```python
from build123d import *

# Parameters (mm, degrees)
F0_W     = 140
F0_H     = 157.3
F0_W_2   = 5.7
F0_H_2   = 42
F0_W_3   = 42
F0_H_3   = 5.7
F0_W_4   = 9.225
F0_H_4   = 11.7
F0_W_5   = 20.361793
F0_H_5   = 125.9
F1_DEPTH = 5.8


with BuildPart() as f1:
    # F0 (on Right) → F1 (new body)
    with BuildSketch(Plane.YZ):
        Rectangle(F0_W, F0_H)
        with Locations((-62.15, -41.3)):
            Rectangle(F0_W_2, F0_H_2, mode=Mode.SUBTRACT)
        with Locations((-32.65, -70.8)):
            Rectangle(F0_W_3, F0_H_3, mode=Mode.SUBTRACT)
        with Locations((-25.8, -41.3)):
            Rectangle(F0_W_2, F0_H_2, mode=Mode.SUBTRACT)
        with Locations((29.475, -70.8)):
            Rectangle(F0_W_3, F0_H_3, mode=Mode.SUBTRACT)
        with Locations((60.0875, -61.45)):
            Rectangle(F0_W_4, F0_H_4, mode=Mode.SUBTRACT)
        with BuildLine():
            ThreePointArc((18.376166, -14.378899), (17.848958, -15.651691), (16.576166, -16.178899))
            Line((16.576166, -16.178899), (2.137455, -16.178901))
            ThreePointArc((2.137455, -16.178901), (0.864663, -15.651693), (0.337455, -14.378901))
            Line((0.337455, -14.378901), (0.337455, 5.028724))
            ThreePointArc((0.337455, 5.028724), (0.864663, 6.301516), (2.137455, 6.828724))
            Line((2.137455, 6.828724), (16.576166, 6.828722))
            ThreePointArc((16.576166, 6.828722), (17.848958, 6.301515), (18.376166, 5.028722))
            Line((18.376166, 5.028722), (18.376166, -1.151716))
            Line((18.376166, -1.151716), (13.94928, -1.151716))
            Line((13.94928, -1.151716), (13.94928, 3.184902))
            Line((13.94928, 3.184902), (4.764341, 3.184902))
            Line((4.764341, 3.184902), (4.764341, -12.535078))
            Line((4.764341, -12.535078), (13.94928, -12.535078))
            Line((13.94928, -12.535078), (13.94928, -7.927517))
            Line((13.94928, -7.927517), (18.376166, -7.927517))
            Line((18.376166, -7.927517), (18.376166, -14.378899))
        make_face(mode=Mode.SUBTRACT)
        Polygon((25.663247, -16.178899), (21.146094, -16.118674), (28.915746, 6.828724), (33.613575, 6.828724), (41.383157, -16.118674), (36.835821, -16.178899), (31.234478, 1.799588), align=None, mode=Mode.SUBTRACT)
        with Locations((-43.830896, 0)):
            Rectangle(F0_W_5, F0_H_5, mode=Mode.SUBTRACT)
        with Locations((-62.15, 41.3)):
            Rectangle(F0_W_2, F0_H_2, mode=Mode.SUBTRACT)
        with Locations((-25.8, 41.3)):
            Rectangle(F0_W_2, F0_H_2, mode=Mode.SUBTRACT)
        with Locations((-32.65, 70.8)):
            Rectangle(F0_W_3, F0_H_3, mode=Mode.SUBTRACT)
        Polygon((3.574371, 9.207119), (0.365742, 9.207119), (0.365742, 20.249205), (3.834504, 20.249205), (6.320433, 14.323433), (8.734065, 20.249205), (12.173907, 20.249205), (12.173907, 9.207119), (9.008657, 9.207119), (9.008657, 14.135599), (7.606707, 9.684005), (4.976251, 9.684005), (3.574371, 14.135599), align=None, mode=Mode.SUBTRACT)
        Polygon((16.899532, 13.571955), (16.899532, 9.207119), (13.633134, 9.207119), (13.633134, 20.249205), (22.536252, 20.249205), (22.536252, 17.589901), (16.899532, 17.589901), (16.899532, 16.086803), (21.264368, 16.086803), (21.264368, 13.571955), align=None, mode=Mode.SUBTRACT)
        Polygon((25.065139, 9.207119), (21.740973, 9.236038), (25.556555, 20.249205), (29.039706, 20.249205), (32.855358, 9.236038), (29.502273, 9.207119), (27.290936, 16.722745), align=None, mode=Mode.SUBTRACT)
        with Locations((29.475, 70.8)):
            Rectangle(F0_W_3, F0_H_3, mode=Mode.SUBTRACT)
        with Locations((60.0875, 61.15)):
            Rectangle(F0_W_4, F0_H_4, mode=Mode.SUBTRACT)
    extrude(amount=F1_DEPTH)


solid = f1.part
```
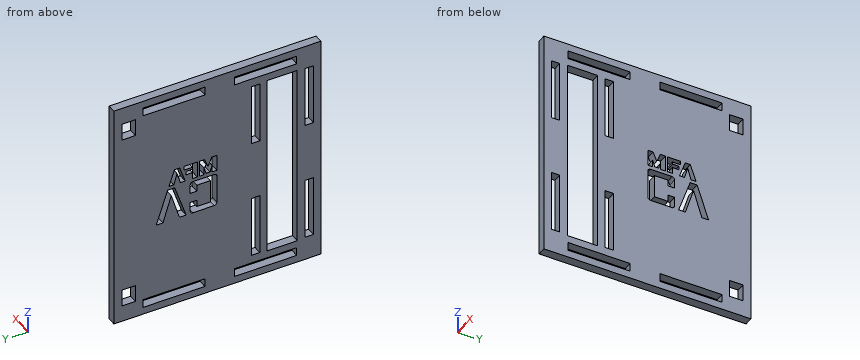
Input: part model. Units: mm. Frame: model coordinates. Give positions to 0.01 mm unless a question says otherwise; leave off trailing zeros. Loops run counter-clockwise (first coordinate to the right, second up) from the corner with the lowest first, then second, coordinate; pieces in that order, holes last.
1) Section query A-A on z = 38.5. Return the cut outline in (x, y).
A:
outline: (0, -70) - (5.8, -70) - (5.8, -65) - (0, -65) - close; (0, -59.3) - (5.8, -59.3) - (5.8, -54.01) - (0, -54.01) - close; (0, -33.65) - (5.8, -33.65) - (5.8, -28.65) - (0, -28.65) - close; (0, -22.95) - (5.8, -22.95) - (5.8, 70) - (0, 70) - close
2) Section query D-D on z = -59.5. Return the cut outline in (x, y) (3 decimals).
A:
outline: (0, -70) - (5.8, -70) - (5.8, -65) - (0, -65) - close; (0, -59.3) - (5.8, -59.3) - (5.8, -54.012) - (0, -54.012) - close; (0, -33.65) - (5.8, -33.65) - (5.8, -28.65) - (0, -28.65) - close; (0, -22.95) - (5.8, -22.95) - (5.8, 55.475) - (0, 55.475) - close; (0, 64.7) - (5.8, 64.7) - (5.8, 70) - (0, 70) - close
3) Section query B-B on y = -51. Return the cut outline in (x, z), and give its area (3 significant figures).
A:
outline: (0, -78.65) - (5.8, -78.65) - (5.8, -73.65) - (0, -73.65) - close; (0, -67.95) - (5.8, -67.95) - (5.8, -62.95) - (0, -62.95) - close; (0, 62.95) - (5.8, 62.95) - (5.8, 67.95) - (0, 67.95) - close; (0, 73.65) - (5.8, 73.65) - (5.8, 78.65) - (0, 78.65) - close
area: 116 mm2
4) Line query: L1, parallel to Z at x = 5.55, y = 2; L2, parallel to Z at x = 2.75, y = -35; L3, parallel to Y at x = 2.35, z = -60 (3 decimals). Output: solid intervals per line, ascending.
A:
L1: z = -78.65 to -16.17, 6.82 to 9.21, 20.25 to 78.65
L2: z = -78.65 to -73.65, -67.95 to -62.95, 62.95 to 67.95, 73.65 to 78.65
L3: y = -70 to -65, -59.3 to -54.012, -33.65 to -28.65, -22.95 to 55.475, 64.7 to 70
5) Section query C-C on y = -16. Return the cut outline in (x, z).
A:
outline: (0, -78.65) - (5.8, -78.65) - (5.8, -73.65) - (0, -73.65) - close; (0, -67.95) - (5.8, -67.95) - (5.8, 67.95) - (0, 67.95) - close; (0, 73.65) - (5.8, 73.65) - (5.8, 78.65) - (0, 78.65) - close
